from build123d import *

# Parameters (mm, degrees)
SKETCH_1_W             = 210
SKETCH_1_H             = 297
EXTRUDE_1_DEPTH        = 0.1
SKETCH_2_W             = 85.6
SKETCH_2_H             = 54
CUT_EXTRUDE_1_DEPTH    = 8
PATTERN_LINEAR_1_COUNT = 3
PATTERN_LINEAR_1_PITCH = 84


with BuildPart() as part:
    # 草图1 → 凸台-拉伸1 (new body)
    with BuildSketch(Plane.XY):
        with Locations((105, 148.5)):
            Rectangle(SKETCH_1_W, SKETCH_1_H)
    extrude(amount=EXTRUDE_1_DEPTH)

    # 草图2 → 切除-拉伸1 (cut)
    with BuildSketch(Plane.XY.offset(0.1)):
        with Locations((105, 64.5)):
            Rectangle(SKETCH_2_W, SKETCH_2_H)
    cut_extrude_1 = extrude(amount=-CUT_EXTRUDE_1_DEPTH, mode=Mode.SUBTRACT)

    # 阵列(线性)1: 切除-拉伸1 ×3
    with Locations(*[(0, i * PATTERN_LINEAR_1_PITCH, 0) for i in range(1, PATTERN_LINEAR_1_COUNT)]):
        add(cut_extrude_1, mode=Mode.SUBTRACT)


solid = part.part
CAD build for the part. Positions are in the model's coordinates, mm. Coordinates: 2 decimals unless noted, no trailing zeros. Order: outer loops, then holes, each group sorted by start corner. A loop starts at its lowest first (then second) coordinate and runs counter-clockwise, first axis right, second up.
Item 1: Band-saw the part on A-A on z = 0.05. List the corners of the cut face in (x, y), plus the area to 3 significant figures.
Check sheet entries:
outline: (0, 0) - (210, 0) - (210, 297) - (0, 297) - close; hole (62.2, 37.5) - (147.8, 37.5) - (147.8, 91.5) - (62.2, 91.5) - close; hole (62.2, 121.5) - (147.8, 121.5) - (147.8, 175.5) - (62.2, 175.5) - close; hole (62.2, 205.5) - (147.8, 205.5) - (147.8, 259.5) - (62.2, 259.5) - close
area: 48,500 mm2
Item 2: Band-saw the part on B-B on x = 134.5. List the corners of the cut face in (y, z).
Check sheet entries:
outline: (0, 0) - (37.5, 0) - (37.5, 0.1) - (0, 0.1) - close; (91.5, 0) - (121.5, 0) - (121.5, 0.1) - (91.5, 0.1) - close; (175.5, 0) - (205.5, 0) - (205.5, 0.1) - (175.5, 0.1) - close; (259.5, 0) - (297, 0) - (297, 0.1) - (259.5, 0.1) - close
Item 3: Band-saw the part on C-C on y = 214. List the corners of the cut face in (x, z), plus the area to 3 significant figures.
Check sheet entries:
outline: (0, 0) - (62.2, 0) - (62.2, 0.1) - (0, 0.1) - close; (147.8, 0) - (210, 0) - (210, 0.1) - (147.8, 0.1) - close
area: 12.4 mm2
Item 4: Drill centre lines: L1, parallel to Y at x = 138, z = 0.05; L2, parallel to X at y = 77, z = 0.05. Where is each one in solid material? Low to high.
Check sheet entries:
L1: y = 0 to 37.5, 91.5 to 121.5, 175.5 to 205.5, 259.5 to 297
L2: x = 0 to 62.2, 147.8 to 210
